Input: part model. Units: mm. Frame: model coordinates. Give positions to 0.01 mm unless a question says otherwise; leave off trailing zeros. Loops run counter-clockwise (first coordinate to the right, second up) from the corner with the lowest first, then second, coordinate; pieces in that order, holes last. Notation, with made-up numbers: M 45.25,-34 L 59.25,-34 A16 cw 59.25,-27 Z; hole C 8.5,-27.5 d1. An arc over 180 degrees is marked long. Return JSON: item names as keys, results as strings. Group by question number.
```python
from build123d import *

# Parameters (mm, degrees)
SKETCH_R          = 1.6
PAD_DEPTH         = 6
SKETCH001_R       = 3
POCKET_DEPTH      = 40.001
POCKET_DEPTH_BACK = 40.001
POCKET001_DEPTH   = 2


with BuildPart() as toolbody:
    # Sketch → Pad (new body)
    with BuildSketch(Plane.XY):
        Polygon((46, -40), (0, -40), (0, -25), (17.5, -25), (0, -7.5), (0, 7.5), (0, 20), (10, 20), (10, 40), (46, 40), (56, 40), (56, -40), align=None)
        with Locations((53, 0)):
            Circle(SKETCH_R, mode=Mode.SUBTRACT)
        with Locations((53, 35)):
            Circle(SKETCH_R, mode=Mode.SUBTRACT)
        with Locations((53, -35)):
            Circle(SKETCH_R, mode=Mode.SUBTRACT)
        with Locations((39, 35)):
            Circle(SKETCH_R, mode=Mode.SUBTRACT)
        with Locations((39, 0)):
            Circle(SKETCH_R, mode=Mode.SUBTRACT)
        with Locations((39, -35)):
            Circle(SKETCH_R, mode=Mode.SUBTRACT)
        with Locations((15, 35)):
            Circle(SKETCH_R, mode=Mode.SUBTRACT)
        with Locations((15, -35)):
            Circle(SKETCH_R, mode=Mode.SUBTRACT)
        Polygon((15, 0), (28.75, 13.75), (28.75, -13.75), align=None, mode=Mode.SUBTRACT)
    extrude(amount=-PAD_DEPTH)

    # Sketch001 → Pocket (cut, two sides)
    with BuildSketch(Plane.XZ) as pocket_sk:
        with Locations((46, 0)):
            Circle(SKETCH001_R)
    extrude(amount=-POCKET_DEPTH, mode=Mode.SUBTRACT)
    extrude(pocket_sk.sketch, amount=POCKET_DEPTH_BACK, mode=Mode.SUBTRACT)

    # Sketch002 (on DatumPlane) → Pocket001 (cut)
    with BuildSketch(Plane.XY.offset(-6)):
        Polygon((16.587713, 32.25), (18.175426, 35), (16.587713, 37.75), (13.412287, 37.75), (11.824574, 35), (13.412287, 32.25), align=None)
        Polygon((40.587713, 32.25), (42.175426, 35), (40.587713, 37.75), (37.412287, 37.75), (35.824574, 35), (37.412287, 32.25), align=None)
        Polygon((54.587713, 32.25), (56.175426, 35), (54.587713, 37.75), (51.412287, 37.75), (49.824574, 35), (51.412287, 32.25), align=None)
        Polygon((54.587713, -2.75), (56.175426, 0), (54.587713, 2.75), (51.412287, 2.75), (49.824574, 0), (51.412287, -2.75), align=None)
        Polygon((40.587713, -2.75), (42.175426, 0), (40.587713, 2.75), (37.412287, 2.75), (35.824574, 0), (37.412287, -2.75), align=None)
        Polygon((54.587713, -37.75), (56.175426, -35), (54.587713, -32.25), (51.412287, -32.25), (49.824574, -35), (51.412287, -37.75), align=None)
        Polygon((40.587713, -37.75), (42.175426, -35), (40.587713, -32.25), (37.412287, -32.25), (35.824574, -35), (37.412287, -37.75), align=None)
        Polygon((16.587713, -37.75), (18.175426, -35), (16.587713, -32.25), (13.412287, -32.25), (11.824574, -35), (13.412287, -37.75), align=None)
    extrude(amount=POCKET001_DEPTH, mode=Mode.SUBTRACT)


with BuildPart() as toolfusion:
    # Part__Mirroring: instance of ToolBody
    add(toolbody.part.mirror(Plane(origin=(0, 0, 0), x_dir=(0, -1, 0), z_dir=(1, 0, 0))))

    # Fusion: union ToolBody
    add(toolbody.part)


solid = toolfusion.part
```
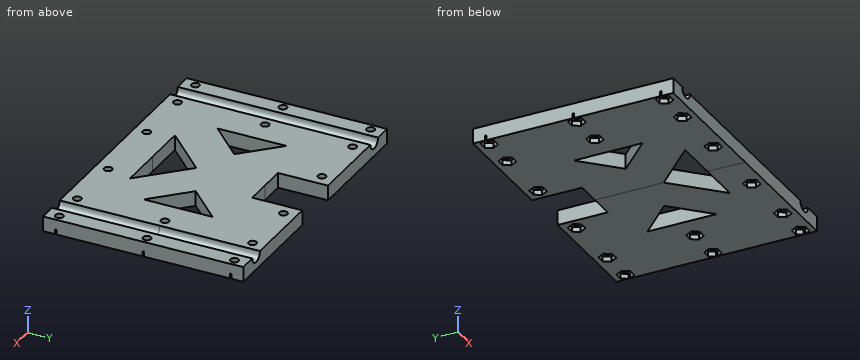
Item 1: First-contact query: pin 1 Ø3.5 at (x, y) = (53, -35) entering from -Z. Flat tip, straight axial feed; report the tip coordinate or a pass-through.
Item 2: Section C-C, the plane y = 26. Return loops of the section in (x, z).
Item 3: Section D-D, the plane x = -46. Return loops of the section in (y, z), then the cut area to 3 significant figures.
Item 4: Section B-B, the plane x = 39. Return loops of the section in (y, z), then the cut area to 3 significant figures.
Item 5: Material intervals for line 1 (X direction, y = 0, z = -4.35); line 2 (Y direction, x = 53, z = -2); line 3 (X direction, y = -8.5, z = -4), sorted ascending. Write a range as from..to.
Item 6: Section A-A, the plane y = -16.5. Return loops of the section in (x, z).
Answer below:
{
 "1": {"pin 1": "z = -4"},
 "2": {"outline": "M -56,-6 L -10,-6 L -10,0 L -43,0 A3 cw -49,0 L -56,0 Z; M 10,-6 L 56,-6 L 56,0 L 49,0 A3 cw 43,0 L 10,0 Z"},
 "3": {"outline": "M -40,-6 L 40,-6 L 40,-3 L -40,-3 Z", "area": "240 mm^2"},
 "4": {"outline": "M -40,-6 L -37.75,-6 L -37.75,-4 L -36.6,-4 L -36.6,0 L -40,0 Z; M -33.4,-4 L -32.25,-4 L -32.25,-6 L -2.75,-6 L -2.75,-4 L -1.6,-4 L -1.6,0 L -33.4,0 Z; M 1.6,-4 L 2.75,-4 L 2.75,-6 L 32.25,-6 L 32.25,-4 L 33.4,-4 L 33.4,0 L 1.6,0 Z; M 36.6,-4 L 37.75,-4 L 37.75,-6 L 40,-6 L 40,0 L 36.6,0 Z", "area": "409 mm^2"},
 "5": {"line 1": "-49.82..-42.18, -35.82..-28.75, -15..15, 28.75..35.82, 42.18..49.82", "line 2": "-40..-36.6, -33.4..-1.6, 1.6..33.4, 36.6..40", "line 3": "-56..-28.75, -23.5..-1, 1..23.5, 28.75..56"},
 "6": {"outline": "M -56,-6 L -9,-6 L -9,0 L -43,0 A3 cw -49,0 L -56,0 Z; M 9,-6 L 56,-6 L 56,0 L 49,0 A3 cw 43,0 L 9,0 Z"}
}
